from build123d import *

# Parameters (mm, degrees)
SKETCH1_R           = 2.5
BOSS_EXTRUDE1_DEPTH = 4


with BuildPart() as part:
    # Sketch1 → Boss-Extrude1 (new body)
    with BuildSketch(Plane.XY):
        Polygon((0, -40), (0, 40), (20, 40), (40, 0), (40, -40), align=None)
        with Locations((10, -29.84)):
            Circle(SKETCH1_R, mode=Mode.SUBTRACT)
        with Locations((30, -29.84)):
            Circle(SKETCH1_R, mode=Mode.SUBTRACT)
        with Locations((10, -9.84)):
            Circle(SKETCH1_R, mode=Mode.SUBTRACT)
        with Locations((10, 10.16)):
            Circle(SKETCH1_R, mode=Mode.SUBTRACT)
        with Locations((10, 30.16)):
            Circle(SKETCH1_R, mode=Mode.SUBTRACT)
        with Locations((30, -9.84)):
            Circle(SKETCH1_R, mode=Mode.SUBTRACT)
    extrude(amount=BOSS_EXTRUDE1_DEPTH)


solid = part.part
Input: part model. Units: mm. Frame: model coordinates. Coordinates: 2 decimals unless noted, no trailing zeros. Order: outer loops, then holes, each group sorted by start corner. A loop starts at its lowest first (then second) coordinate and runs counter-clockwise, first axis right, second up.
1. Cut plane D-D, the plane x = 30. Return loops of the section in (y, z).
Checked values:
outline: (-40, 0) - (-32.34, 0) - (-32.34, 4) - (-40, 4) - close; (-27.34, 0) - (-12.34, 0) - (-12.34, 4) - (-27.34, 4) - close; (-7.34, 0) - (20, 0) - (20, 4) - (-7.34, 4) - close
2. Cut plane C-C, the plane y = -29.84. Return loops of the section in (x, z), plus the area to 3 significant figures.
Checked values:
outline: (0, 0) - (7.5, 0) - (7.5, 4) - (0, 4) - close; (12.5, 0) - (27.5, 0) - (27.5, 4) - (12.5, 4) - close; (32.5, 0) - (40, 0) - (40, 4) - (32.5, 4) - close
area: 120 mm2
3. Cut plane B-B, the plane y = 10.16. Return loops of the section in (x, z).
Checked values:
outline: (0, 0) - (7.5, 0) - (7.5, 4) - (0, 4) - close; (12.5, 0) - (34.92, 0) - (34.92, 4) - (12.5, 4) - close
4. Draft query along X for faces 1 (the flat face through (10, 40, 2)), 2 (the cylindrical face through (9.67, -7.36, 1.97)), 3 (the flat face through (40, -20, 2)). Return one class per face: +X half, -X half, draft (parallel to the pull), parting line (faces both ways), or undercut.
Checked values:
face 1: draft
face 2: undercut
face 3: +X half
5. Contact query for a flat-ended pin moving along its axis: P1, Ø1.5, axis at y = 15.5, z = 1, coming from the +X side (3 decimals). Output: stop coordinate, or through.
Checked values:
P1: stops at x = 32.625
6. Cut plane A-A, the plane x = 10. Return loops of the section in (y, z).
Checked values:
outline: (-40, 0) - (-32.34, 0) - (-32.34, 4) - (-40, 4) - close; (-27.34, 0) - (-12.34, 0) - (-12.34, 4) - (-27.34, 4) - close; (-7.34, 0) - (7.66, 0) - (7.66, 4) - (-7.34, 4) - close; (12.66, 0) - (27.66, 0) - (27.66, 4) - (12.66, 4) - close; (32.66, 0) - (40, 0) - (40, 4) - (32.66, 4) - close
7. Ray query, line 1 along Y through (x, z) = (10, 2.8); line 2 along X through (y, z) = (-30, 3.7); line 3 along Y through (x, z) = (30, 3.15). Return the intervals inside material, ascending.
Checked values:
line 1: y = -40 to -32.34, -27.34 to -12.34, -7.34 to 7.66, 12.66 to 27.66, 32.66 to 40
line 2: x = 0 to 7.51, 12.49 to 27.51, 32.49 to 40
line 3: y = -40 to -32.34, -27.34 to -12.34, -7.34 to 20
